Design review of the part built by this model. Coordinates are the model's own, in mm. Face numbers are marked on the shaded views. A direction names the side the tool comes from. Give positions to 0.01 mm unless a question says otherwise; leave off trailing zeros. Loops run counter-clockwise (first coordinate to the right, second up) from the corner with the lowest first, then second, coordinate; pieces in that order, holes last. Notation, with made-up numbers: (13.25, 60.25) -> (69.25, 60.25) arc R19 ccw to (69.25, 78.25) -> close; hole circle Ø5 at (45.25, 85.5). An arc over 180 degrees is marked (long way). Use a Markdown table: item, result. Add a question column.
1. Draft analysis for pull direction X (two halves, no side actions). For the marked faces 3, 4 and 5, state which applies: pulls with the +X half, pulls with the -X half, needs draft (parallel to the pull), parting line crosses it, or undercut.
2. Add section A-A (y = 10). State the section outline as (x, z) points.
3. Add section C-C (x = 31.5). State the section outline as (y, z) points.
4. For the marked faces 1 and 2, list the 3-axis set-ups (+Z, -Z, +X, -X, +Y, -Y) from which the entire face can be reached by the end or side of a thin tool; tool diameter is ignored.
5. To check wall thickness, follow line 1 (Y direction, x = -37.45, z = 0.6); line 2 (Y direction, x = 37.55, z = 1.15); line 3 (Y direction, x = -21.93, z = 1.35). State the ranges of each line that lie inside material, in increasing order.
6. Add section B-B (z = 3.25). State the section outline as (x, y) points.
7. For pin 1 Ø1 at (y, z) = (9, 6.5) entering from -X; pin 2 Ø2 at (x, z) = (5, 4) entering from -Y; pin 3 Ø0.6 at (x, z) = (8.5, 8.5) entering from +Y; pin 4 Ø1 at (x, y) = (-9.43, 15.67) entering from +Z, all flat-tipped, find the tip position at first contact; note any pin that passes through.
8. Add section D-D (z = 7). State the section outline as (x, y) points, and give its area (3 significant figures).
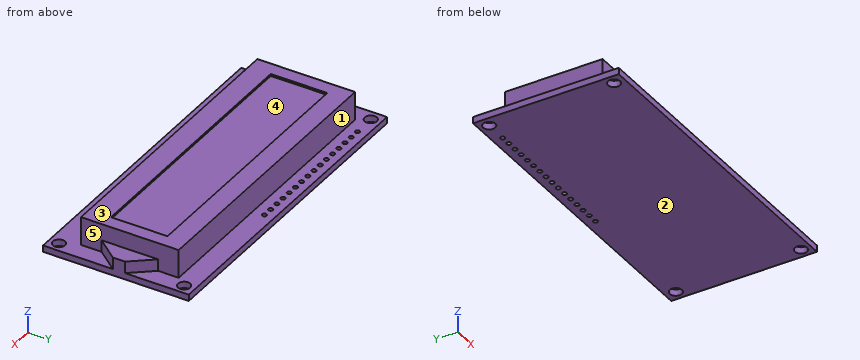
```python
from build123d import *

# Parameters (mm, degrees)
F0_W     = 80
F0_H     = 36.1
F0_R     = 1.5
F0_R_2   = 0.55
F1_DEPTH = 1.6
F3_DEPTH = 7
F4_DEPTH = 2.9
F5_W     = 64.5
F5_H     = 14
F6_DEPTH = 0.5


with BuildPart() as f1:
    # F0 (on Top) → F1 (new body)
    with BuildSketch(Plane.XY):
        Rectangle(F0_W, F0_H)
        with Locations((-37.55, -15.4)):
            Circle(F0_R, mode=Mode.SUBTRACT)
        with Locations((37.55, -15.6)):
            Circle(F0_R, mode=Mode.SUBTRACT)
        with Locations((-37.45, 15.6)):
            Circle(F0_R, mode=Mode.SUBTRACT)
        with Locations((-31.93, 15.67)):
            Circle(F0_R_2, mode=Mode.SUBTRACT)
        with Locations((-29.43, 15.67)):
            Circle(F0_R_2, mode=Mode.SUBTRACT)
        with Locations((-26.93, 15.67)):
            Circle(F0_R_2, mode=Mode.SUBTRACT)
        with Locations((-24.43, 15.67)):
            Circle(F0_R_2, mode=Mode.SUBTRACT)
        with Locations((-21.93, 15.67)):
            Circle(F0_R_2, mode=Mode.SUBTRACT)
        with Locations((-19.43, 15.67)):
            Circle(F0_R_2, mode=Mode.SUBTRACT)
        with Locations((-16.93, 15.67)):
            Circle(F0_R_2, mode=Mode.SUBTRACT)
        with Locations((-14.43, 15.67)):
            Circle(F0_R_2, mode=Mode.SUBTRACT)
        with Locations((-11.93, 15.67)):
            Circle(F0_R_2, mode=Mode.SUBTRACT)
        with Locations((-9.43, 15.67)):
            Circle(F0_R_2, mode=Mode.SUBTRACT)
        with Locations((-6.93, 15.67)):
            Circle(F0_R_2, mode=Mode.SUBTRACT)
        with Locations((-4.43, 15.67)):
            Circle(F0_R_2, mode=Mode.SUBTRACT)
        with Locations((-1.93, 15.67)):
            Circle(F0_R_2, mode=Mode.SUBTRACT)
        with Locations((0.57, 15.67)):
            Circle(F0_R_2, mode=Mode.SUBTRACT)
        with Locations((3.07, 15.67)):
            Circle(F0_R_2, mode=Mode.SUBTRACT)
        with Locations((5.57, 15.67)):
            Circle(F0_R_2, mode=Mode.SUBTRACT)
        with Locations((37.55, 15.4)):
            Circle(F0_R, mode=Mode.SUBTRACT)
    extrude(amount=F1_DEPTH)

    # F2 (on face) → F3 (join)
    with BuildSketch(Plane.XY.offset(1.6)):
        Polygon((-35.6, 12.85), (-35.6, -11.35), (35.6, -11.35), (35.6, -6.25), (35.6, 7.75), (35.6, 12.85), align=None)
    extrude(amount=F3_DEPTH)

    # F2 (on face) → F4 (join)
    with BuildSketch(Plane.XY.offset(1.6)):
        Polygon((-35.6, 12.85), (-35.6, -11.35), (35.6, -11.35), (35.6, -6.25), (35.6, 7.75), (35.6, 12.85), align=None)
        Polygon((35.6, 7.75), (35.6, -6.25), (40, -0.75), (40, 2.25), align=None)
    extrude(amount=F4_DEPTH)

    # F5 (on face) → F6 (cut)
    with BuildSketch(Plane.XY.offset(8.6)):
        with Locations((0.05, 1.05)):
            Rectangle(F5_W, F5_H)
    extrude(amount=-F6_DEPTH, mode=Mode.SUBTRACT)


solid = f1.part
```
Taken from the geometry:
| question | item | result |
|---|---|---|
| 1 | face 3 | needs draft |
| 1 | face 4 | undercut |
| 1 | face 5 | pulls with the +X half |
| 2 | outline | (-40, 0) -> (40, 0) -> (40, 1.6) -> (35.6, 1.6) -> (35.6, 8.6) -> (-35.6, 8.6) -> (-35.6, 1.6) -> (-40, 1.6) -> close |
| 3 | outline | (-18.05, 0) -> (18.05, 0) -> (18.05, 1.6) -> (12.85, 1.6) -> (12.85, 8.6) -> (8.05, 8.6) -> (8.05, 8.1) -> (-5.95, 8.1) -> (-5.95, 8.6) -> (-11.35, 8.6) -> (-11.35, 1.6) -> (-18.05, 1.6) -> close |
| 4 | face 1 | +Z, +X, -X, +Y |
| 4 | face 2 | -Z, +X, -X, +Y, -Y |
| 5 | line 1 | y = -18.05 to -16.9, -13.9 to 14.1, 17.1 to 18.05 |
| 5 | line 2 | y = -18.05 to -17.1, -14.1 to 13.9, 16.9 to 18.05 |
| 5 | line 3 | y = -18.05 to 15.12, 16.22 to 18.05 |
| 6 | outline | (-35.6, -11.35) -> (35.6, -11.35) -> (35.6, -6.25) -> (40, -0.75) -> (40, 2.25) -> (35.6, 7.75) -> (35.6, 12.85) -> (-35.6, 12.85) -> close |
| 7 | pin 1 | stops at x = -35.6 |
| 7 | pin 2 | stops at y = -11.35 |
| 7 | pin 3 | stops at y = 12.85 |
| 7 | pin 4 | passes through |
| 8 | outline | (-35.6, -11.35) -> (35.6, -11.35) -> (35.6, 12.85) -> (-35.6, 12.85) -> close |
| 8 | area | 1,720 mm^2 |
